Autodesk Inventor part; units mm, degrees
ref_plane "Work Plane1" through (-30, 20, 6.5) normal (-1, 0, 0) x (0, 0, 1)
ref_plane "Work Plane2" through (-54, 110, 6.5) normal (0, 1, 0) x (1, 0, 0)
ref_plane "YZ Plane" through (0, 0, 0) normal (1, 0, 0) x (0, 1, 0)
sketch "Sketch1" plane through (0, 0, 0) normal (0, 0, 1) x (1, 0, 0)
  line L0 (0, 0) -> (-60, 0)
  line L1 (-60, 0) -> (-60, 20)
  line L2 (-60, 20) -> (-60, 110)
  line L3 (-60, 110) -> (-30, 110)
  line L4 (-30, 0) -> (-30, 110)
  line L5 (-30, 20) -> (-55.65, 20)
  line L6 (-55.65, 20) -> (-55.65, 85)
  line L7 (-55.65, 85) -> (-30, 85)
  line L8 (0, 20) -> (0, 110)
  line L9 (0, 110) -> (-30, 110)
  line L10 (-30, 20) -> (-4.35, 20)
  line L11 (-4.35, 20) -> (-4.35, 85)
  line L12 (-4.35, 85) -> (-30, 85)
  line L13 (0, 0) -> (0, 20)
  line L14 (-30, 20) -> (-45, 20)
  dimension "d0" = 60
  dimension "d1" = 20
  dimension "d2" = 90
  dimension "d3" = 65
  dimension "d39" = 15
extrude "Extrusion1" add sketch "Sketch1" along normal mid plane 13 contours L0 L4 L10 L11 L12 L9 L8 L13 | L0 L1 L2 L3 L4 L7 L6 L5
sketch "Sketch2" plane through (0, 0, 6.5) normal (1, 0, 0) x (0, 0, -1)
  line L0 (13, 0) -> (13, 110)
  line L1 (13, 0) -> (13, 20)
  line L2 (13, 20) -> (36.3, 20)
  line L3 (36.3, 20) -> (13, 110)
  point P0 (6.5, 0)
  dimension "d6" = 20
  dimension "d7" = 23.3
extrude "Extrusion2" add sketch "Sketch2" against normal blind 22
ref_plane "Work Plane1" through (-30, 20, 6.5) normal (-1, 0, 0) x (0, 0, 1)
mirror "Mirror1" about plane through (-30, 20, 6.5) normal (-1, 0, 0) of "Extrusion2"
sketch "Sketch3" plane through (0, 0, 6.5) normal (0, 0, 1) x (1, 0, 0)
  line L0 (-4.35, 20) -> (-55.65, 20)
  line L1 (-30, 20) -> (-30, 0)
  line L2 (-60, 0) -> (0, 0)
  line L3 (-30, 16.1731) -> (-45.5, 16.1731)
  line L4 (-30, 16.1731) -> (-14.5, 16.1731)
  dimension "d17" = 15.5
sketch "Sketch4" plane through (0, 0, 6.5) normal (0, 0, 1) x (1, 0, 0)
  line L0 (-55.65, 85) -> (-4.35, 85)
  line L1 (-30, 85) -> (-30, 110)
  line L2 (0, 110) -> (-60, 110)
  line L3 (-30, 85) -> (-30, 90)
  line L4 (-30, 90) -> (-30, 105)
  point P0 (0, 0)
  dimension "d25" = 5
  dimension "d26" = 15
hole "Hole2" at (-30, 90, 6.5) at (-30, 105, 6.5) direction (0, 0, -1) diameter 3.242 end through all
sketch "Sketch5" plane through (-60, 20, -29.8) normal (0, -1, 0) x (1, 0, 0)
  line L0 (0, 0) -> (22, 0)
  line L1 (0, 0) -> (0, 6)
  line L2 (0, 0) -> (0, 23.3)
  line L3 (0, 6) -> (60, 6)
  line L4 (60, 0) -> (60, 23.3)
  line L5 (60, 6) -> (43, 6)
  line L6 (0, 6) -> (17, 6)
  point P0 (60, 29.8)
  point P1 (17, 6)
  dimension "d34" = 6
  dimension "d35" = 17
  dimension "d36" = 17
hole "Hole3" at (-43, 20, -23.8) at (-17, 20, -23.8) direction (0, 1, 0) diameter 3 end through all
sketch "Sketch6" plane through (0, 0, 6.5) normal (1, 0, 0) x (0, 0, -1)
  line L0 (13, 110) -> (0, 110)
  line L1 (13, 0) -> (13, 20)
  line L2 (13, 110) -> (13, 20)
  line L3 (36.3, 20) -> (13, 20)
  line L4 (13, 20) -> (36.3, 20)
  line L5 (13, 110) -> (36.3, 20)
  line L6 (36.3, 20) -> (13, 110)
  point P0 (6.5, 0)
extrude "Extrusion3" cut sketch "Sketch6" against normal blind 12
mirror "Mirror2" about plane through (-30, 20, 6.5) normal (-1, 0, 0) of "Extrusion3"
sketch "Sketch8" plane through (0, 0, 6.5) normal (0, 0, 1) x (1, 0, 0)
  line L0 (-4.35, 20) -> (-55.65, 20)
  line L1 (-30, 20) -> (-30, 85)
  line L2 (-55.65, 85) -> (-4.35, 85)
  line L3 (-30, 20) -> (-37, 20)
  line L4 (-37, 20) -> (-37, 85)
  line L5 (-55.65, 20) -> (-55.65, 85)
  line L6 (-37, 85) -> (-55.65, 85)
  line L7 (-55.65, 85) -> (-55.65, 20)
  line L8 (-55.65, 20) -> (-37, 20)
  line L9 (-23, 20) -> (-23, 85)
  line L10 (-4.35, 20) -> (-4.35, 85)
  line L11 (-23, 85) -> (-4.35, 85)
  line L12 (-4.35, 85) -> (-4.35, 20)
  line L13 (-4.35, 20) -> (-23, 20)
  point P0 (0, 0)
  point P1 (-23, 85)
  dimension "d43" = 7
extrude "Extrusion5" add sketch "Sketch8" against normal blind 13 contours L0 L9 L2 L10 | L0 L5 L2 L4
sketch "Sketch9" plane through (-60, 0, 6.5) normal (0, -1, 0) x (1, 0, 0)
  line L0 (60, -13) -> (60, 0)
  line L1 (60, 0) -> (0, 0)
  line L2 (60, -13) -> (0, -13)
  line L3 (0, -13) -> (0, 0)
  line L4 (0, 0) -> (60, 0)
  line L5 (60, 0) -> (60, -13)
  point P0 (60, -6.5)
extrude "Extrusion6" cut sketch "Sketch9" against normal blind 8
fillet "Fillet1" radius 6 4 edges at (0, 8, 0) (-60, 8, 0) (-60, 110, 0) (0, 110, 0)
fillet "Fillet2" radius 4 2 edges at (-48, 65, -6.5) (-12, 65, -6.5)
ref_plane "Work Plane2" through (-54, 110, 6.5) normal (0, 1, 0) x (1, 0, 0)
sketch "Sketch10" plane through (-54, 110, 6.5) normal (0, 1, 0) x (1, 0, 0)
  circle A0 centre (11, 30.3) radius 1.5
  line L0 (11, 30.3) -> (11, 36.3)
  line L1 (6, 36.3) -> (16, 36.3)
  circle A1 centre (37, 30.3) radius 1.5
  line L2 (37, 30.3) -> (37, 36.3)
  line L3 (42, 36.3) -> (32, 36.3)
  point P0 (54, 6.5)
hole "Hole4" at (-43, 110, -23.8) at (-17, 110, -23.8) direction (0, -1, 0) diameter 7 depth 85
hole "Hole5" at (-14.5, 16.1731, 6.5) at (-45.5, 16.1731, 6.5) direction (0, 0, -1) diameter 2.4 end through all
thread "Thread1"
thread "Thread2"
properties part number "stand_less_rough"
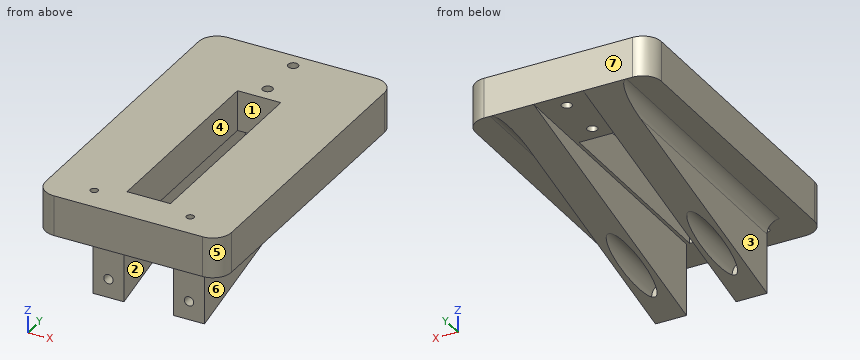
Input: part model. Units: mm. Frame: model coordinates. Face numbers are marked on the shaded views. A direction names the side the tool comes from. Give positions to 0.01 mm unless a question says otherwise; leave off trailing zeros. Loops run counter-clockwise (first coordinate to the right, second up) from the corner with the lowest first, then second, coordinate; pieces in that order, holes last. Notation, with made-up numbers: M 86,29.5 L 123,29.5 A14 cw 123,33.5 Z; hole C -31.5,73 d9. An arc over 180 degrees is marked long. Use one line per item in the form item = value.
1. Section query D-D, the plane y = 90. Return the cut outline in (x, z).
Numbers:
outline = M -60,-6.5 L -52,-6.5 A4 cw -48,-10.5 L -48,-11.68 L -38,-11.68 L -38,-6.5 L -31.62,-6.5 L -31.62,6.5 L -60,6.5 Z; M -28.38,-6.5 L -22,-6.5 L -22,-11.68 L -12,-11.68 L -12,-10.5 A4 cw -8,-6.5 L 0,-6.5 L 0,6.5 L -28.38,6.5 Z
2. Section query B-B, the plane x = -24.5. Return the cut outline in (y, z).
Numbers:
outline = M 8,-6.5 L 20,-6.5 L 20,6.5 L 8,6.5 Z; M 85,-6.5 L 110,-6.5 L 110,6.5 L 85,6.5 Z
3. First-contact query: pin 1 (1 mm diameter, centred on y = 56, z = -19, fed in from +X); pin 2 (4 mm diameter, centred on x = -22, y = 96, fed in from -Z); pin 3 (4 mm diameter, centred on x = -46, z = -17.5, fed in from -Y); pin 4 (2.5 mm diameter, centred on x = -17, z = -23.8, fed in from -Y). Flat tips, straight axial feed; report the tip coordinate or a pass-through.
Numbers:
pin_1 = -12
pin_2 = -10.64
pin_3 = 20
pin_4 = through
4. Section query C-C, the plane z = -7.5. Return the cut outline in (x, y), and give its area (3 significant figures).
Numbers:
outline = M -49.35,20 L -38,20 L -38,106.14 L -49.35,106.14 Z; M -22,20 L -10.65,20 L -10.65,106.14 L -22,106.14 Z
area = 1,960 mm²
5. Line query: L1, parallel to X at y = 22, z = -23.8; L2, parallel to X at y = 33, z = 1; L3, parallel to Y at x = -14.5, z = 1.75. Output: solid intervals per line, ascending.
Numbers:
L1 = -48 to -44.5, -41.5 to -38, -22 to -18.5, -15.5 to -12
L2 = -60 to -37, -23 to 0
L3 = 8 to 14.97, 17.37 to 110
6. Section query A-A, the plane y = 29. Return the cut outline in (x, z).
Numbers:
outline = M -60,-6.5 L -52,-6.5 A4 cw -48,-10.5 L -48,-27.47 L -38,-27.47 L -38,-6.5 L -37,-6.5 L -37,6.5 L -60,6.5 Z; M -23,-6.5 L -22,-6.5 L -22,-27.47 L -12,-27.47 L -12,-10.5 A4 cw -8,-6.5 L 0,-6.5 L 0,6.5 L -23,6.5 Z; hole C -43,-23.8 d7; hole C -17,-23.8 d7
7. Pull-direction query (Y, two-part tool) for the marked faces 4, 5, 6 and 7; classes: released by +Y, released by -Y, zero draft, split by the parting line, or undercut.
Numbers:
face_4 = undercut
face_5 = released by -Y
face_6 = zero draft
face_7 = released by +Y
8. Reachability of the marked faces 1, 2 and 3 from +Z, -Z, +X, -X, +Y, -Y: full face, straight path, thin tool, end or side. Return the list, or none.
Numbers:
face_1 = +Z, -Z
face_2 = -Z, +Y, -Y
face_3 = -Z, -X, +Y, -Y
